Autodesk Inventor part; units mm, degrees
ref_plane "YZ Plane" through (0, 0, 0) normal (1, 0, 0) x (0, 1, 0)
ref_plane "XZ Plane" through (0, 0, 0) normal (0, 1, 0) x (-1, 0, 0)
ref_plane "XY Plane" through (0, 0, 0) normal (0, 0, 1) x (1, 0, 0)
sketch "Sketch1" plane through (0, 0, 0) normal (0, 1, 0) x (-1, 0, 0)
  circle A0 centre (0, 0) radius 3
  dimension "d0" = 6
extrude "Extrusion1" add sketch "Sketch1" along normal blind 3
sketch "Sketch2" plane through (0, 3, 0) normal (0, 1, 0) x (1, 0, 0)
  circle A0 centre (0, 0) radius 1.5
  dimension "d3" = 3
extrude "Extrusion2" add sketch "Sketch2" along normal blind 20
thread "Thread1"
chamfer "Chamfer1" distance 0.5 angle 45 1 edges at (-1.5, 23, 0)
properties part number "reverse gear link stud"
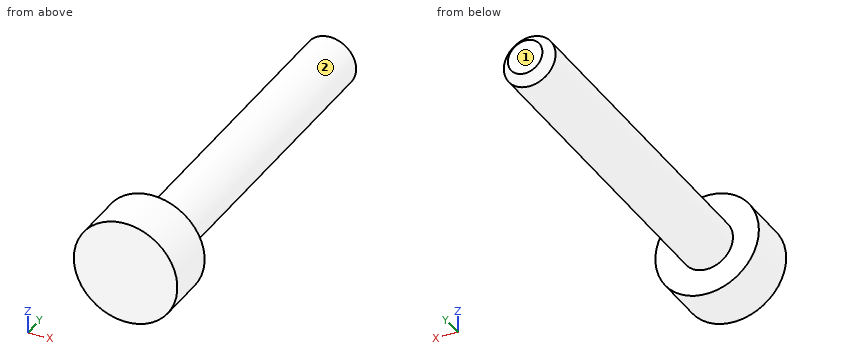
Geometry check sheet. Reference: the model listing, model coordinates, mm. Face numbers are marked on the shaded views. A direction names the side the tool comes from. Give positions to 0.01 mm unless a question says otherwise; leave off trailing zeros. Loops run counter-clockwise (first coordinate to the right, second up) from the corner with the lowest first, then second, coordinate; pieces in that order, holes last. Notation, with made-up numbers: M -9,-5 L 36,-5 A26 ccw 36,30 Z; hole C 78.5,80 d2. An arc over 180 degrees is marked long. Write item = value, one per line.
(1) Sectioned sample at D-D, the plane y = 1.5. Record the cut outline in (x, z).
Answer below:
outline = C 0,0 d6
(2) Material ranges on line 1 (Y direction, x = -1.5, z = -2.4); line 2 (X direction, y = 6.25, z = -0.1); line 3 (Z direction, x = -0.95, y = 3.75), recorded low to high. Write a range as [from, to].
Answer below:
line_1 = [0, 3]
line_2 = [-1.5, 1.5]
line_3 = [-1.16, 1.16]
(3) Gauge pin test, flat ends, axial feed: pin 1 Ø2 at (y, z) = (7, -2) entering from -X; pin 2 Ø3 at (y, z) = (11, -1) entering from -X; pin 3 Ø2 at (x, y) = (0, 13.5) entering from +Z. Record the tip position at first contact, or that the pin passes through.
Answer below:
pin_1 = -1.12
pin_2 = -1.5
pin_3 = 1.5
(4) Sectioned sample at C-C, the plane y = 12. Record the cut outline in (x, z), plus the area to 3 significant figures.
Answer below:
outline = C 0,0 d3
area = 7.07 mm2
(5) Sectioned sample at A-A, the plane x = 0. Record the cut outline in (y, z), plus the area to 4 significant figures.
Answer below:
outline = M 0,-3 L 3,-3 L 3,-1.5 L 22.5,-1.5 L 23,-1 L 23,1 L 22.5,1.5 L 3,1.5 L 3,3 L 0,3 Z
area = 77.75 mm2
(6) Tool access check on the marked faces 1 and 2. Record the directions out of +Z, -Z, +X, -X, +Y, -Y that give a thin tool (end or side, any length) a straight path to the whole face; none if there is none.
Answer below:
face_1 = +Z, -Z, +X, -X, +Y
face_2 = +Y
(7) Sectioned sample at B-B, the plane z = 0. Record the cut outline in (x, y), plus the area to 4 significant figures.
Answer below:
outline = M -3,0 L 3,0 L 3,3 L 1.5,3 L 1.5,22.5 L 1,23 L -1,23 L -1.5,22.5 L -1.5,3 L -3,3 Z
area = 77.75 mm2
